```python
from build123d import *

# Parameters (mm, degrees)
BOSS_EXTRUDE1_DEPTH = 20
SKETCH2_W           = 30
SKETCH2_H           = 6
BOSS_EXTRUDE2_DEPTH = 3


with BuildPart() as part:
    # Sketch1 → Boss-Extrude1 (new body)
    with BuildSketch(Plane(origin=(0, 0, 0), x_dir=(0, 0, -1), z_dir=(1, 0, 0))):
        Polygon((-9.8, -12.38), (-3.8, -12.38), (-3.8, -3.357082066), (0, 0), (-5.1, 0), (-5.1, 37.9), (-0.3, 37.9), (-0.3, 41), (-9.8, 41), align=None)
    extrude(amount=BOSS_EXTRUDE1_DEPTH)

    # Sketch2 → Boss-Extrude2 (add)
    with BuildSketch(Plane.XZ.offset(12.38)):
        with Locations((10, 6.8)):
            Rectangle(SKETCH2_W, SKETCH2_H)
    extrude(amount=-BOSS_EXTRUDE2_DEPTH)


solid = part.part
```
For this review, take the finished solid that the model builds, in its own axes (mm). A direction names the side the tool comes from. Give positions to 0.01 mm unless a question says otherwise; leave off trailing zeros. Write each loop counter-clockwise with the first axis right and the second up, starting at its lowest first coordinate (ties: lowest second). Pieces come first, ordered by that corner, then holes. Notation, with made-up numbers: M -18.75,58 L -1.75,58 A23 ccw -1.75,84 Z; hole C -27.5,74.25 d3. An arc over 180 degrees is marked long. Answer as a JSON object with one key per item and string values. Group by question number.
Item 1: Consider section D-D on y = 2. Write out the cut boundary in (x, z), plus the area to 3 significant figures.
Item 2: For probe 1 along Y at (x, z) = (17.5, 4); probe 2 along X at (y, z) = (15, 9.25); probe 3 along Y at (x, z) = (-0.5, 8.5), list the stretches that pass through material, from the lowest coordinate up. Write a range as [from, to].
Item 3: Consider section A-A on z = 1.75. Write out the cut boundary in (x, y).
Item 4: Draft analysis for pull direction Y (two halves, no side actions). For faces 4 (the flat face through (10, 39, 0.3)), 5 (the flat face through (10, 19, 5.1)), 6 (the flat face through (10, 41, 5)), state which applies: +Y half, -Y half, draft (parallel to the pull), parting line (faces both ways), or undercut.
Item 5: Consider section B-B on x = 9.75. Write out the cut boundary in (y, z).
Item 6: Consider section C-C on z = 6.25. Write out the cut boundary in (x, y).
Item 7: For pin 1 Ø1 at (y, z) = (26, 8.5) entering from -X; pin 2 Ø10 at (x, y) = (9, 20.5) entering from -Z; pin 3 Ø5 at (y, z) = (22.5, 4) entering from +X; pin 4 Ø5.5 at (x, z) = (6, 2) entering from -Y, all flat-tipped, find the tip position at first contact; note any pin that passes through.
Item 8: Tool access review of faces 1 (the flat face through (22, -9.38, 7)), 2 (the flat face through (0, 16, 7)), 3 (the flat face through (10, 0, 3)): name each direction out of +Z, -Z, +X, -X, +Y, -Y from which nothing blocks a thin tool from reaching the whole face with its end or side.
Check result:
{
 "1": {"outline": "M 0,5.1 L 20,5.1 L 20,9.8 L 0,9.8 Z", "area": "94.0 mm^2"},
 "2": {"probe 1": "y = [-12.38, 0], [37.9, 41]", "probe 2": "x = [0, 20]", "probe 3": "y = [-12.38, -9.38]"},
 "3": {"outline": "M 0,-1.55 L 20,-1.55 L 20,0 L 0,0 Z; M 0,37.9 L 20,37.9 L 20,41 L 0,41 Z"},
 "4": {"face 4": "draft", "face 5": "undercut", "face 6": "+Y half"},
 "5": {"outline": "M -12.38,3.8 L -3.36,3.8 L 0,0 L 0,5.1 L 37.9,5.1 L 37.9,0.3 L 41,0.3 L 41,9.8 L -12.38,9.8 Z"},
 "6": {"outline": "M -5,-12.38 L 25,-12.38 L 25,-9.38 L 20,-9.38 L 20,41 L 0,41 L 0,-9.38 L -5,-9.38 Z"},
 "7": {"pin 1": "stops at x = 0", "pin 2": "stops at z = 5.1", "pin 3": "stops at x = 20", "pin 4": "stops at y = -12.38"},
 "8": {"face 1": "+Z, -Z, +X, +Y", "face 2": "+Z, -Z, -X, +Y", "face 3": "-Z, +X, -X"}
}
